CAD build for the part. Positions are in the model's coordinates, mm. Round coordinates to 2 decimals unless told otherwise and drop trailing zeros. Loops run counter-clockwise (first coordinate to the right, second up) from the corner with the lowest first, then second, coordinate; pieces in that order, holes last. Notation, with made-up numbers: (-36.75, -11) - (-24.75, -11) arc R30 cw to (-24.75, 11) - close; hole circle Ø8 at (-15.75, -32). An arc over 180 degrees is marked (long way). Use one line per item in the form item = value.
Autodesk Inventor part; units mm, degrees
ref_plane "Work Plane1" through (0, 0, 0) normal (0, 0, 1) x (1, 0, 0)
ref_plane "YZ Plane" through (0, 0, 0) normal (1, 0, 0) x (0, 1, 0)
ref_plane "XZ Plane" through (0, 0, 0) normal (0, 1, 0) x (-1, 0, 0)
ref_plane "Work Plane1" through (0, 0, 0) normal (0, 0, 1) x (1, 0, 0)
sketch "Sketch1" plane through (0, 0, 0) normal (0, 0, 1) x (1, 0, 0)
  circle A0 centre (31.2751, 14.3567) radius 2.032
  circle A1 centre (-31.2751, -10.7579) radius 2.032
  circle A2 centre (-9.1964, -21.5433) radius 2.032
  line L0 (4.4799, 27.3609) -> (32.7659, 20.5292)
  arc A3 (4.4799, 27.3609) -> (-15.0435, 20.5211) centre (0.0075, 8.8433) ccw
  line L1 (-36.2921, -6.8653) -> (-15.0435, 20.5211)
  arc A4 (-36.2921, -6.8653) -> (-27.8312, -16.0929) centre (-31.2751, -10.7579) ccw
  arc A5 (-19.0523, -17.9839) -> (-27.8312, -16.0929) centre (-24.3873, -21.4279) ccw
  line L2 (-14.5314, -24.9873) -> (-19.0523, -17.9839)
  arc A6 (36.9334, 11.4747) -> (32.7659, 20.5292) centre (31.2751, 14.3567) ccw
  arc A7 (-14.5314, -24.9873) -> (-5.9915, -27.0252) centre (-9.1964, -21.5433) ccw
  arc A8 (25.6029, -8.5539) -> (28.0563, -5.954) centre (22.398, -3.072) ccw
  circle A9 centre (22.398, -3.072) radius 2.032
  line L3 (36.9334, 11.4747) -> (28.0563, -5.954)
  line L4 (25.6029, -8.5539) -> (-5.9915, -27.0252)
  line L5 (72.5061, 7.5054) -> (72.5061, 11.8054)
  circle A10 centre (0.0075, 8.8433) radius 2.2225
  point P0 (0, 0)
  dimension "d14" = 4.064
  dimension "d17" = 4.445
extrude "Plate3" add sketch "Sketch1" along normal blind 1.5875 contours L0 A6 L3 A8 L4 A7 L2 A5 A4 L1 A3 | A10
sketch "Sketch2" plane through (0, 0, 1.5875) normal (0, 0, 1) x (1, 0, 0)
  arc A0 (4.4799, 27.3609) -> (-15.0435, 20.5211) centre (0.0075, 8.8433) ccw
  line L0 (4.4799, 27.3609) -> (32.7659, 20.5292)
  arc A1 (36.9334, 11.4747) -> (32.7659, 20.5292) centre (31.2751, 14.3567) ccw
  line L1 (36.9334, 11.4747) -> (28.0563, -5.954)
  arc A2 (25.6029, -8.5539) -> (28.0563, -5.954) centre (22.398, -3.072) ccw
  line L2 (25.6029, -8.5539) -> (-5.9915, -27.0252)
  arc A3 (-14.5314, -24.9873) -> (-5.9915, -27.0252) centre (-9.1964, -21.5433) ccw
  line L3 (-14.5314, -24.9873) -> (-19.0523, -17.9839)
  arc A4 (-19.0523, -17.9839) -> (-27.8312, -16.0929) centre (-24.3873, -21.4279) ccw
  arc A5 (-36.2921, -6.8653) -> (-27.8312, -16.0929) centre (-31.2751, -10.7579) ccw
  line L4 (-36.2921, -6.8653) -> (-15.0435, 20.5211)
  circle A6 centre (31.2751, 14.3567) radius 2.032
  circle A7 centre (22.398, -3.072) radius 2.032
  circle A8 centre (-9.1964, -21.5433) radius 2.032
  circle A9 centre (-31.2751, -10.7579) radius 2.032
  circle A10 centre (0.0075, 8.8433) radius 2.2225
  point P0 (0, 0)
  dimension "d16" = 4.445
extrude "Extrusion1" cut sketch "Sketch2" against normal blind 15.875 contours A10
equation "\"d15\" = Thickness"
equation "\"BendRadius\" = Thickness"
equation "\"BendReliefWidth\" = Thickness"
equation "\"BendReliefDepth\" = 0.5 * Thickness"
equation "\"CornerReliefSize\" = 4 * Thickness"
equation "\"MinimumRemnant\" = 2 * Thickness"
equation "\"TransitionRadius\" = BendRadius"
equation "\"JacobiRadiusSize\" = BendRadius"
equation "\"GapSize\" = Thickness"
properties part number "Front Horizontal Odom Pod Rot Side" material "Acetal Resin, White"
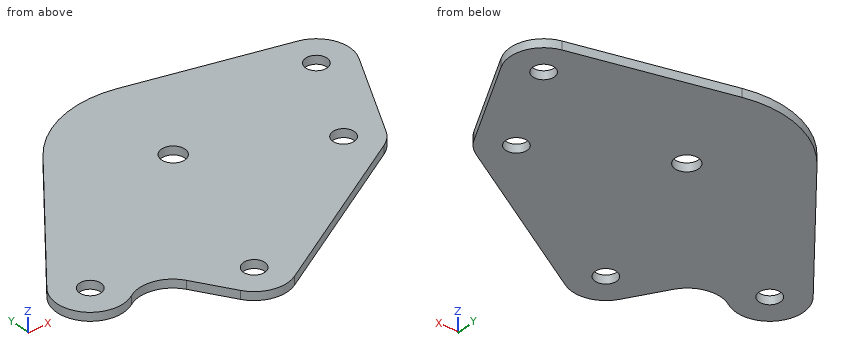
1) Slice it at C-C (x = 31.5). Write the cut outline in (y, z), plus the area to 3 significant figures.
Report:
outline = (0.81, 0) - (12.34, 0) - (12.34, 1.59) - (0.81, 1.59) - close; (16.38, 0) - (20.83, 0) - (20.83, 1.59) - (16.38, 1.59) - close
area = 25.4 mm^2
2) Drill centre lines: probe 1 along X at (y, z) = (-9, 0.7); probe 2 along Y at (x, z) = (24, 0.3); probe 3 along Y at (x, z) = (-30.5, 1). Where is each one in solid material? Low to high.
Report:
probe_1 = -37.38 to -32.29, -30.26 to 24.84
probe_2 = -9.49 to -4.32, -1.82 to 22.65
probe_3 = -17.06 to -12.64, -8.88 to 0.6
3) Slice it at A-A (x = -9.5). Write the cut outline in (y, z).
Report:
outline = (-27.89, 0) - (-23.55, 0) - (-23.55, 1.59) - (-27.89, 1.59) - close; (-19.53, 0) - (25.35, 0) - (25.35, 1.59) - (-19.53, 1.59) - close
4) Slice it at D-D (y = 1). Write the cut outline in (x, z), plus the area to 3 significant figures.
Report:
outline = (-30.19, 0) - (31.6, 0) - (31.6, 1.59) - (-30.19, 1.59) - close
area = 98.1 mm^2
5) Slice it at B-B (z = 1.2). Write the cut outline in (x, y) (1 decimal), plus the area to 3 significant figures.
Report:
outline = (-36.3, -6.9) arc R6.4 ccw to (-27.8, -16.1) arc R6.3 cw to (-19.1, -18) - (-14.5, -25) arc R6.3 ccw to (-6, -27) - (25.6, -8.6) arc R6.3 ccw to (28.1, -6) - (36.9, 11.5) arc R6.3 ccw to (32.8, 20.5) - (4.5, 27.4) arc R19.1 ccw to (-15, 20.5) - close; hole circle Ø4.1 at (-31.3, -10.8); hole circle Ø4.1 at (-9.2, -21.5); hole circle Ø4.4 at (0, 8.8); hole circle Ø4.1 at (22.4, -3.1); hole circle Ø4.1 at (31.3, 14.4)
area = 2,520 mm^2
6) Flat gauge pins, fed straight in: pin 1 (6.5 mm diameter, centred on x = -31.28, y = -10.76, fed in from +Z); pin 2 (3.5 mm diameter, centred on x = 22.398, y = -3.072, fed in from -Z). Where does each tip first touch, or does it go through?
Report:
pin_1 = 1.59
pin_2 = through
